CAD build for the part. Positions are in the model's coordinates, mm. Give positions to 0.01 mm unless a question says otherwise; leave off trailing zeros. Write each loop counter-clockwise with the first axis right and the second up, starting at its lowest first coordinate (ties: lowest second). Pieces come first, ordered by that corner, then holes. Notation, with made-up numbers: (53, 26) - (91, 26) arc R17 ccw to (91, 43) - close; hole circle Ø3 at (21.25, 53). An arc over 180 degrees is marked (long way). Answer as a JSON object with one key per item and string values.
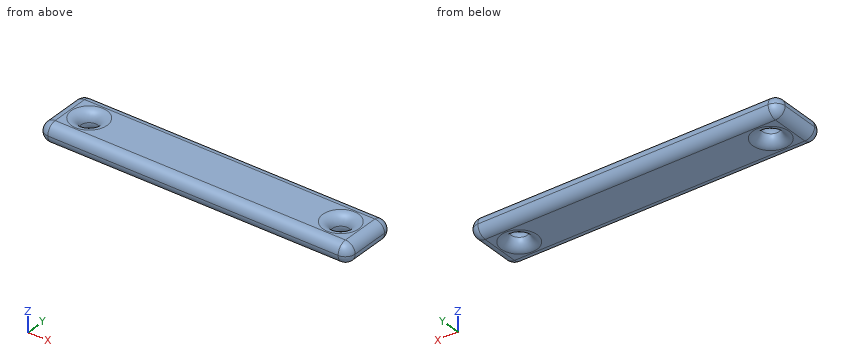
from build123d import *

# Parameters (mm, degrees)
SKETCH_1_W      = 64
SKETCH_1_H      = 12
SKETCH_1_R      = 1.7
EXTRUDE_1_DEPTH = 2
FILLET_1_R      = 2


with BuildPart() as part:
    # 草图1 → 凸台-拉伸1 (new, symmetric)
    with BuildSketch(Plane.XY):
        with Locations((26, 0)):
            Rectangle(SKETCH_1_W, SKETCH_1_H)
        Circle(SKETCH_1_R, mode=Mode.SUBTRACT)
        with Locations((52, 0)):
            Circle(SKETCH_1_R, mode=Mode.SUBTRACT)
    extrude(amount=EXTRUDE_1_DEPTH, both=True)

    # 圆角1
    fillet_1_edges = [part.edges().sort_by_distance(p)[0] for p in [
        (-1.7, 0, -2),
        (-1.7, 0, 2),
        (-6, 0, 2),
        (50.3, 0, -2),
        (50.3, 0, 2),
        (26, -6, 2),
        (58, 0, 2),
        (26, -6, -2),
        (-6, 0, -2),
        (26, 6, -2),
        (58, 0, -2),
        (58, -6, 0),
        (-6, -6, 0),
        (-6, 6, 0),
        (58, 6, 0),
        (26, 6, 2),
    ]]
    fillet(fillet_1_edges, radius=FILLET_1_R - 0.0001)  # a hair under: the kernel refuses the full size


solid = part.part
(1) Flat gauge pins, fed straight in: P1, Ø4.5, axis at x = 52, y = 0, coming from the -Z side; P2, Ø2, axis at x = 1, y = -2, coming from the -Z side; P3, Ø2, axis at x = 0, y = 0, coming from the -Z side. Where does each tip first touch, or does it go through?
Answer key:
{"P1": "stops at z = -1.38", "P2": "stops at z = -1.95", "P3": "passes through"}
(2) Probe L1, parallel to X at y = 0, z = 0.05; L2, parallel to Y at x = 52, z = 0; L3, parallel to X at y = 0.75, z = 0.35. List the from-to ranges inside material, lowest first. Write a range as [from, to].
Answer key:
{"L1": "x = [-6, -1.7], [1.7, 50.3], [53.7, 58]", "L2": "y = [-6, -1.7], [1.7, 6]", "L3": "x = [-5.97, -1.56], [1.56, 50.44], [53.56, 57.97]"}
(3) Saw through at B-B, the plane y = 0. State how many separate pieces and enclosed holes the cut face has, and give its area (4 significant figures).
Answer key:
{"separate pieces": "3", "enclosed holes": "0", "area": "218.5 mm²"}
(4) Saw through at D-D, the plane z = -1.4. Give the cut face in (x, y).
Answer key:
{"outline": "(-5.43, -4) arc R1.43 ccw to (-4, -5.43) - (56, -5.43) arc R1.43 ccw to (57.43, -4) - (57.43, 4) arc R1.43 ccw to (56, 5.43) - (-4, 5.43) arc R1.43 ccw to (-5.43, 4) - close; hole circle Ø4.54 at (0, 0); hole circle Ø4.54 at (52, 0)"}
